```python
from build123d import *

# Parameters (mm, degrees)
F1_DEPTH = 25.4
F2_SIZE  = 25.4
F3_R     = 6.35
F4_R     = 3.175
F5_R     = 4.05
F6_DEPTH = 25.4010001


with BuildPart() as f1:
    # F0 (on Right) → F1 (new body)
    with BuildSketch(Plane.YZ):
        Polygon((-177.8, 0), (0, 0), (0, 177.8), (-25.3918121044, 177.8), (-25.3918121044, 12.7), (-137.4, 12.7), (-132.4, 25.4), (-142.4, 25.4), (-147.4, 12.7), (-172.8, 12.7), (-167.8, 25.4), (-177.8, 25.4), align=None)
    extrude(amount=F1_DEPTH)

    # F2
    f2_edges = [f1.edges().sort_by_distance(p)[0] for p in [
        (12.7, -25.391812, 12.7),
    ]]
    chamfer(f2_edges, length=F2_SIZE)

    # F3
    f3_edges = [f1.edges().sort_by_distance(p)[0] for p in [
        (12.7, 0, 0),
        (12.7, 0, 177.8),
        (12.7, -25.391812, 177.8),
        (12.7, -177.8, 25.4),
        (12.7, -177.8, 0),
    ]]
    fillet(f3_edges, radius=F3_R)

    # F4
    f4_edges = [f1.edges().sort_by_distance(p)[0] for p in [
        (12.7, -172.8, 12.7),
        (12.7, -137.4, 12.7),
        (12.7, -147.4, 12.7),
        (12.7, -142.4, 25.4),
        (12.7, -132.4, 25.4),
        (12.7, -167.8, 25.4),
        (12.7, -25.391812, 38.1),
        (12.7, -50.791812, 12.7),
    ]]
    fillet(f4_edges, radius=F4_R)

    # F5 (on face) → F6 (cut, through all)
    with BuildSketch(Plane.YZ.offset(25.4)):
        with Locations((-12.7061052421, 161.9854427668)):
            Circle(F5_R)
        with Locations((-12.8001880162, 16.1035214467)):
            Circle(F5_R)
    extrude(amount=-F6_DEPTH, mode=Mode.SUBTRACT)


solid = f1.part
```
Work out the finished part from the listing and answer in its coordinate system (mm). A direction names the side the tool comes from. Coordinates: 2 decimals unless noted, no trailing zeros. Write each loop counter-clockwise with the first axis right and the second up, starting at its lowest first coordinate (ties: lowest second). Pieces come first, ordered by that corner, then holes.
Q1. Each of these flat-tipped pins is pushed along its axis until it touches: pin 1 Ø3 at (x, y) = (4.5, -140) entering from +Z; pin 2 Ø12.5 at (x, z) = (13, 131) entering from -Y; pin 3 Ø1.5 at (x, y) = (16, -54) entering from +Z. Where does it stop, or does it pass through?
Q2. Determine the mould class of faces 4 (the face through (25.4, -23, 56)), 5 (the face through (12.88, -175.89, 1.81)), 6 (the face through (13, -92, 12.7)) for opening direction Y: released by +Y, released by -Y, zero draft, split by the parting line, or undercut.
Q3. A cutting plane is placed at A-A, the plane y = -121.5. Give the vertices of the cut face in (x, z), then the cut area to 3 significant figures.
Q4. A cutting plane is placed at C-C, the plane x = 5.25. State how many separate pieces and enclosed holes the cut face has, then the cut area to 3 significant figures.
Q5. Find the intervals of material crossed by line 1 (Y direction, x = 6.75, z = 14); line 2 (Z direction, x = 18.25, y = -91); line 3 (Y direction, x = 15.25, z = 44), in increasing order.
Q6. Which of the six approach directions +Z, -Z, +X, -X, +Y, -Y give full straight-line access (tool end or side, diameter ignored) to faces 1 (the face through (13, -177.8, 13)), 2 (the face through (12.522, -170.348, 18.927)), 3 (the face through (13, -159, 12.7))?
Q7. A cutting plane is placed at B-B, the plane z = 95. Give the vertices of the cut face in (x, y).
Findings below:
1. pin 1: stops at z = 25.4
1. pin 2: stops at y = -25.39
1. pin 3: stops at z = 12.7
2. face 4: zero draft
2. face 5: released by -Y
2. face 6: undercut
3. outline: (0, 0) - (25.4, 0) - (25.4, 12.7) - (0, 12.7) - close
3. area: 323 mm2
4. separate pieces: 1
4. enclosed holes: 2
4. area: 6,850 mm2
5. line 1: y = -177.8 to -170.7, -147 to -135.3, -49.49 to -16.26, -9.34 to 0
5. line 2: z = 0 to 12.7
5. line 3: y = -25.39 to 0
6. face 1: +Z, -Z, +X, -X, -Y
6. face 2: +X, -X
6. face 3: +Z, +X, -X
7. outline: (0, -25.39) - (25.4, -25.39) - (25.4, 0) - (0, 0) - close
